The drawing under review shows one solid part. Ordinate dimensions are in mm from its lowest x, y, z. A direction names the side the tool comes from. Round coordinates to 2 decimals unless told otherwise and drop trailing zeros. Order: outer loops, then holes, each group sorted by start corner. A loop starts at its lowest first (then second) coordinate and runs counter-clockwise, first axis right, second up. Notation, with made-up numbers: (63, 37.25) -> (76, 37.25) arc R37 cw to (76, 74.25) -> close; hole circle Ø9 at (18, 31). An arc over 180 degrees is marked (long way). Use a Markdown table: item, result. Add a question column.
1) Clearance check with flat-ended pins moving along their axes: P1, Ø9, axis at x = 26, z = 6, coming from the +Y side; P2, Ø4.5, axis at y = 9.2, z = 20, coming from the -X side; P3, Ø7, axis at y = 41.2, z = 20, coming from the -X side; P4, Ø6, axis at x = 9.5, y = 7.5, coming from the +Z side. State where each tip first meets the part, or that it passes through.
2) Machinability: for the marked faces 1, 2 and 3, which of the approach directions +Z, -Z, +X, -X, +Y, -Y give a long, thin tool a straight path to every point of the face, cutting with its end or side? Answer none if there is none.
3) Consider section C-C (z = 6). State the section outline as (x, y) points.
4) Wall thickness on line 1 along Y through (x, z) = (49.75, 20); line 2 along Y through (x, z) = (8, 3.75); line 3 along X through (y, z) = (13.5, 4): over which ranges is each line inside the solid? List them lowest first. Write a range as [from, to].
5) Consider section D-D (z = 14). State the section outline as (x, y) points.
6) Consider section A-A (y = 41.2). State the section outline as (x, z) points.
7) Consider section B-B (x = 34). State the section outline as (y, z) points.
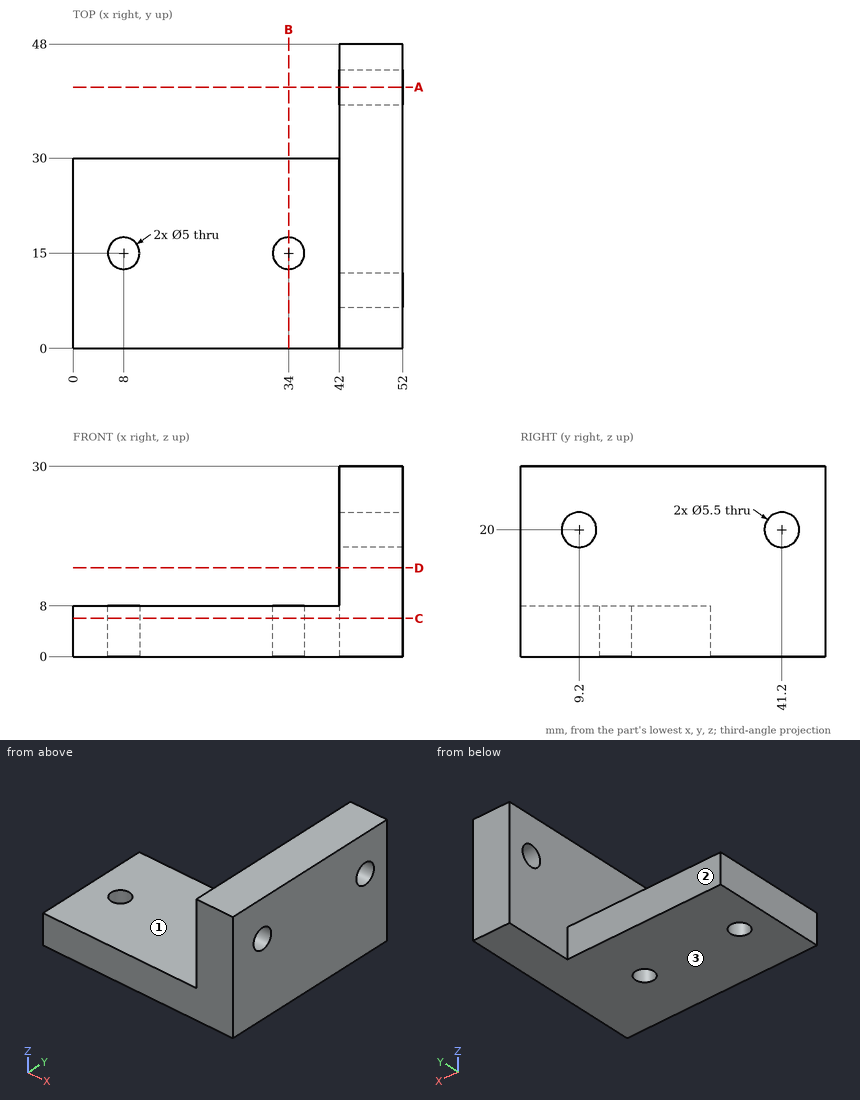
Results list:
| question | item | result |
|---|---|---|
| 1 | P1 | y = 30 |
| 1 | P2 | through |
| 1 | P3 | x = 42 |
| 1 | P4 | z = 8 |
| 2 | face 1 | +Z, -X, +Y, -Y |
| 2 | face 2 | +Z, -Z, -X, +Y |
| 2 | face 3 | -Z, +X, -X, +Y, -Y |
| 3 | outline | (0, 0) -> (52, 0) -> (52, 48) -> (42, 48) -> (42, 30) -> (0, 30) -> close; hole circle Ø5 at (8, 15); hole circle Ø5 at (34, 15) |
| 4 | line 1 | [0, 6.45], [11.95, 38.45], [43.95, 48] |
| 4 | line 2 | [0, 12.5], [17.5, 30] |
| 4 | line 3 | [0, 6], [10, 32], [36, 52] |
| 5 | outline | (42, 0) -> (52, 0) -> (52, 48) -> (42, 48) -> close |
| 6 | outline | (42, 0) -> (52, 0) -> (52, 17.25) -> (42, 17.25) -> close; (42, 22.75) -> (52, 22.75) -> (52, 30) -> (42, 30) -> close |
| 7 | outline | (0, 0) -> (12.5, 0) -> (12.5, 8) -> (0, 8) -> close; (17.5, 0) -> (30, 0) -> (30, 8) -> (17.5, 8) -> close |
